Autodesk Inventor part; units mm, degrees
ref_plane "YZ Plane" through (0, 0, 0) normal (1, 0, 0) x (0, 1, 0)
ref_plane "XZ Plane" through (0, 0, 0) normal (0, 1, 0) x (-1, 0, 0)
ref_plane "XY Plane" through (0, 0, 0) normal (0, 0, 1) x (1, 0, 0)
sketch "Skizze6" plane through (0, 0, 0) normal (0, 1, 0) x (-1, 0, 0)
  line L0 (69, 0) -> (158, 0)
  line L1 (158, 0) -> (158, 16)
  line L2 (0, 30) -> (0, 8)
  line L3 (0, 8) -> (69, 8)
  line L4 (69, 8) -> (69, 0)
  line L5 (0, 30) -> (75, 30)
  line L6 (75, 30) -> (158, 16)
  point P0 (0, 0)
  dimension "d34" = 89
  dimension "d35" = 22
  dimension "d36" = 30
  dimension "d37" = 158
  dimension "d38" = 75
  dimension "d41" = 16
extrude "Extrusion2" add sketch "Skizze6" along normal blind 10
sketch "Skizze7" plane through (0, 10, 0) normal (0, 1, 0) x (1, 0, 0)
  line L0 (-69, 0) -> (-158, 0)
  line L1 (-158, 0) -> (-158, -16)
  point P0 (0, 0)
  point P1 (-138, -8)
  point P2 (-113.5, -8)
  point P3 (-89, -8)
  point P4 (-138.2626, -14.3361)
  dimension "d42" = 8
  dimension "d43" = 20
  dimension "d44" = 24.5
  dimension "d45" = 24.5
hole "Bohrung5" at (-113.5, 10, 8) at (-89, 10, 8) at (-138, 10, 8) direction (0, -1, 0) diameter 5.5 end through all
sketch "Skizze8" plane through (0, 0, 0) normal (0, -1, 0) x (1, 0, 0)
  arc A0 (-12.5, 21.25) -> (-12.5, 16.75) centre (-12.5, 19) ccw
  line L0 (-75, 30) -> (0, 30)
  arc A1 (-7.5, 16.75) -> (-7.5, 21.25) centre (-7.5, 19) ccw
  line L1 (-7.5, 16.75) -> (-12.5, 16.75)
  line L2 (-7.5, 21.25) -> (-12.5, 21.25)
  line L3 (0, 30) -> (0, 8)
  line L4 (-158, 0) -> (-158, 16)
  point P0 (0, 0)
  dimension "d53" = 4.5
  dimension "d54" = 11
  dimension "d55" = 4.5
  dimension "d56" = 5
  dimension "d58" = 145.5
extrude "Extrusion3" cut sketch "Skizze8" against normal through all
fillet "Rundung1" radius 5 6 edges at (-69, 5, 8) (-69, 5, 0) (0, 5, 8) (0, 5, 30) (-158, 5, 16) (-158, 5, 0)
fillet "Rundung2" radius 300 1 edges at (-75, 5, 30)
properties part number "106.016.01_Anbindung_Vereinzelung"
Geometry: final body of the model. Coordinates: model frame, mm. A direction names the side the tool comes from. Round coordinates to 2 decimals unless told otherwise and drop trailing zeros. Order: outer loops, then holes, each group sorted by start corner. A loop starts at its lowest first (then second) coordinate and runs counter-clockwise, first axis right, second up. Notation, with made-up numbers: M 44,26 L 97,26 A21 ccw 97,45 Z; hole C 37.5,66 d10. An arc over 180 degrees is marked long. Use one line per item in the form item = value. Start each with the question number.
Q1. Cut plane D-D (x = -38.5). Return loops of the section in (y, z), and give its area (3 significant figures).
Q2. Pin query (flat end, axial travel): pin 1 Ø4 at (x, y) = (-9, 4) entering from -Z; pin 2 Ø2 at (x, y) = (-111, 4) entering from +Z; pin 3 Ø1 at (x, y) = (-101.5, 2) entering from +Z. Return the tip coordinate at first contact, or that it passes through.
Q3. Cut plane A-A (x = -138). Return loops of the section in (y, z), and give its area (3 significant figures).
Q4. Mould query, pull axis Z, two halves, no side actions, for faces 3 (the face through (-156.85, 5.07, 14.96)), 4 (the face through (-14.75, 4.93, 19.05)), 5 (the face through (-156, 5, 1)). Classes: +Z half, -Z half, draft (parallel to the pull), parting line (faces both ways), or undercut.
Q5. Material intervals for line 1 (X direction, y = 6, z = 8.5); line 2 (Z direction, x = -39.5, y = 4); line 3 (Z direction, x = -113.5, y = 6), sorted ascending. Write a range as [from, to].
Q6. Access query for faces 1 (the face through (0, 5, 19)), 2 (the face through (-5.25, 4.93, 18.95)). Directions: +Z, -Z, +X, -X, +Y, -Y. A direction counts if a zero-diameter tool reaches every point of the face in a straight line with its end or side. Return the directions, or none.
Q7. Cut plane C-C (x = -113.5). Return loops of the section in (y, z), and give its area (3 significant figures).
Q8. Cut plane B-B (y = 3.5). Count the separate pieces of the cut face and the enclosed holes in it, and give its area (3 significant figures).
Geometry results:
q1.outline = M 0,8 L 10,8 L 10,30 L 0,30 Z
q1.area = 220 mm^2
q2.pin_1 = 8
q2.pin_2 = 24.1
q2.pin_3 = 25.61
q3.outline = M 0,0 L 10,0 L 10,5.25 L 0,5.25 Z; M 0,10.75 L 10,10.75 L 10,19.37 L 0,19.37 Z
q3.area = 139 mm^2
q4.face_3 = +Z half
q4.face_4 = undercut
q4.face_5 = -Z half
q5.line_1 = [-158, -140.7], [-135.3, -116.2], [-110.8, -91.7], [-86.3, -2.82]
q5.line_2 = [8, 30]
q5.line_3 = [0, 5.25], [10.75, 23.51]
q6.face_1 = +Z, -Z, +X, +Y, -Y
q6.face_2 = +Y, -Y
q7.outline = M 0,0 L 10,0 L 10,5.25 L 0,5.25 Z; M 0,10.75 L 10,10.75 L 10,23.51 L 0,23.51 Z
q7.area = 180 mm^2
q8.separate_pieces = 1
q8.enclosed_holes = 4
q8.area = 3,460 mm^2
